Could you check a few things on this drawing? It's one solid part, dimensions in mm from its lowest x, y, z. A direction names the side the tool comes from. Round coordinates to 2 decimals unless told otherwise and drop trailing zeros. Write each loop counter-clockwise with the first axis right and the second up, starting at its lowest first coordinate (ties: lowest second). Pieces come first, ordered by that corner, then holes. Notation, with made-up numbers: (-15.75, 63) -> (8.25, 63) arc R30 cw to (8.25, 97) -> close; hole circle Ø2 at (11, -40). An arc over 180 degrees is marked (long way). Answer in a Markdown table with one row per item.
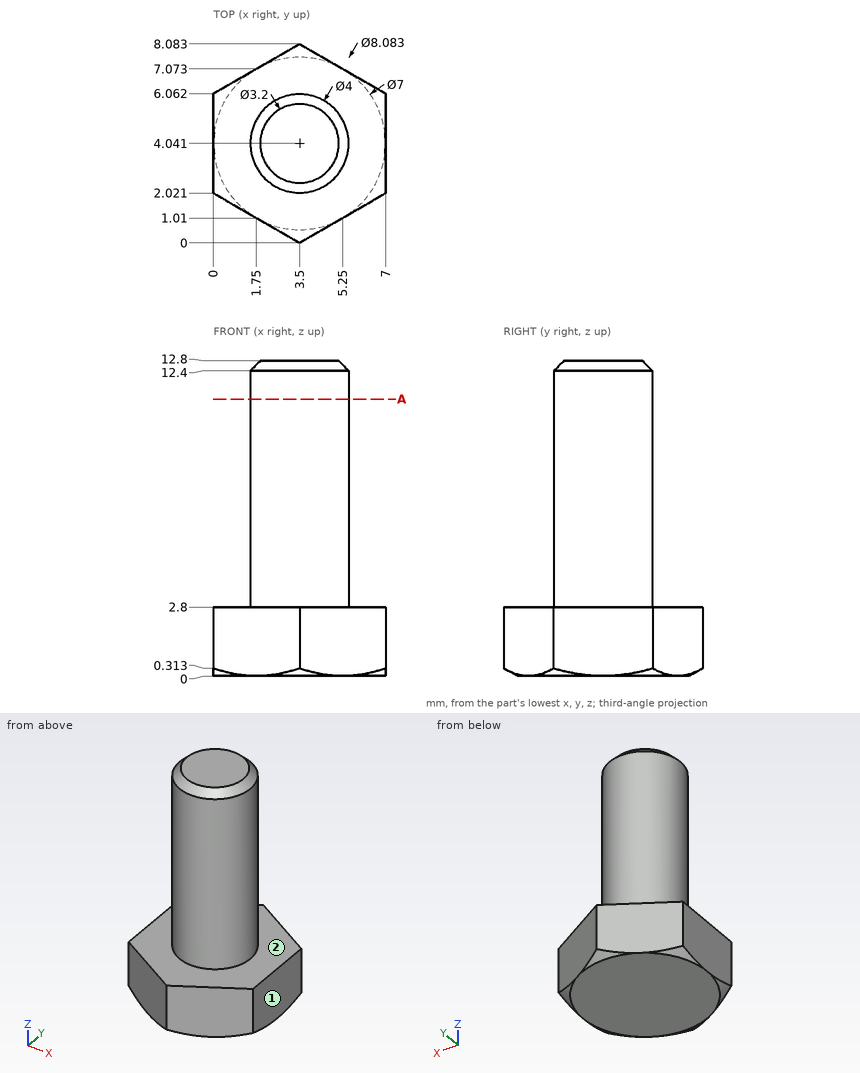
1) Please list where these lines run through material, in increasing order: line 1 (Z direction, x = 1.5, y = 2); line 2 (Y direction, x = 6.5, z = 1); line 3 (X direction, y = 5, z = 7.5) (1 decimal).
Findings:
| item | result |
|---|---|
| line 1 | z = 0 to 2.8 |
| line 2 | y = 1.73 to 6.35 |
| line 3 | x = 1.7 to 5.3 |
2) For pin 1 (3 mm diameter, centred on x = 3, z = 10.5, fed in from -Y), with a flat end and sliding along its axis, tell me the tip position at first contact or that it passes through.
Findings:
| item | result |
|---|---|
| pin 1 | stops at y = 2.04 |
3) For the marked faces 1 and 2, which set-ups out of +Z, -Z, +X, -X, +Y, -Y let a thin tool reach every point of the face, with its end or its side?
Findings:
| item | result |
|---|---|
| face 1 | +Z, -Z, +X, +Y, -Y |
| face 2 | +Z |
4) Imagine slicing it at A-A, the plane z = 11.25. Please give me the cut outline in (x, y).
Findings:
| item | result |
|---|---|
| outline | circle Ø4 at (3.5, 4.04) |
